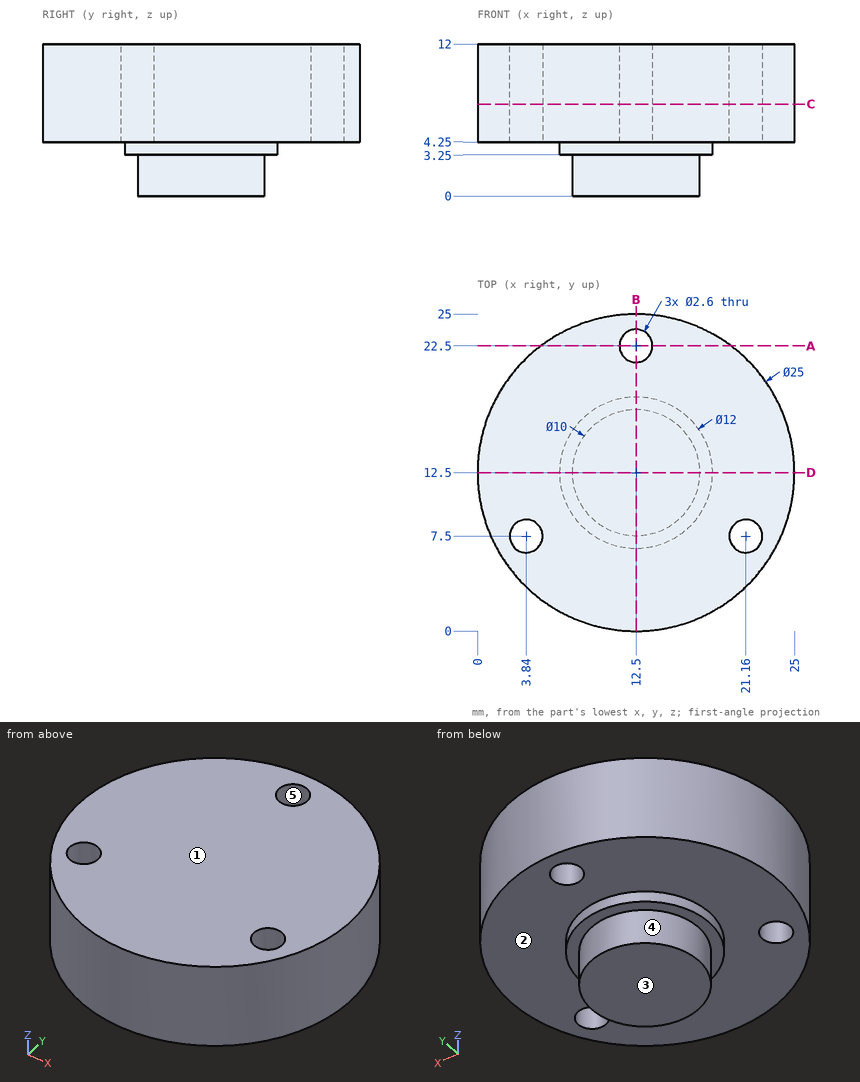
Part print with two shaded views. Sizes in mm from the minimum x, y, z corner. A direction names the side the tool comes from. Round coordinates to 2 decimals unless told otherwise and drop trailing zeros. Order: outer loops, then holes, each group sorted by start corner. A loop starts at its lowest first (then second) coordinate and runs counter-clockwise, first axis right, second up. Notation, with made-up numbers: (2.5, 71) - (56.5, 71) arc R18 ccw to (56.5, 97) - close; hole circle Ø10 at (70, 67.5). An arc over 180 degrees is marked (long way). Answer as CSV lines item,"result". Start each with the question number.
1. Drill centre lines: L1, parallel to Y at x = 12.5, z = 7.75; L2, parallel to Z at x = 15.5, y = 20; L3, parallel to Y at x = 11.5, z = 11.25. Where is each one in solid material? Low to high. Write a range as [from, to].
2. Tool access for the marked faces 1 and 2: list every direction of +Z, -Z, +X, -X, +Y, -Y with a clear straight run to the whole face (end or side of a thin tool).
3. Pin check, flat tips, straight feed: pin 1 (1.5 mm diameter, centred on y = 10, z = 3, fed in from -X); pin 2 (2.5 mm diameter, centred on x = 3.84, y = 7.5, fed in from -Z); pin 3 (1.5 mm diameter, centred on x = 6.5, z = 10.5, fed in from -Y); pin 4 (1.5 mm diameter, centred on x = 17, y = 18.5, fed in from -Z). Stop position of each tip, or through.
4. Saw through at A-A, the plane y = 22.5. Write the cut outline in (x, z).
5. Saw through at D-D, the plane y = 12.5. Write the cut outline in (x, z).
6. Saw through at C-C, the plane z = 7.25. Write the cut outline in (x, y), and give its area (3 significant figures).
7. Pull direction X, two halves, no side cores. Call the marked faces 3, 4 and 5: +X half, -X half, draft (parallel to the pull), parting line (faces both ways), or undercut.
8. Saw through at B-B, the plane x = 12.5. Write the cut outline in (y, z), and give its area (3 significant figures).
Model answer:
1,L1,"y = [0, 21.2], [23.8, 25]"
1,L2,"z = [4.25, 12]"
1,L3,"y = [0.04, 21.67], [23.33, 24.96]"
2,face 1,"+Z, +X, -X, +Y, -Y"
2,face 2,"-Z"
3,pin 1,"stops at x = 6.77"
3,pin 2,"passes through"
3,pin 3,"stops at y = 1.16"
3,pin 4,"stops at z = 4.25"
4,outline,"(5, 4.25) - (11.2, 4.25) - (11.2, 12) - (5, 12) - close; (13.8, 4.25) - (20, 4.25) - (20, 12) - (13.8, 12) - close"
5,outline,"(0, 4.25) - (6.5, 4.25) - (6.5, 3.25) - (7.5, 3.25) - (7.5, 0) - (17.5, 0) - (17.5, 3.25) - (18.5, 3.25) - (18.5, 4.25) - (25, 4.25) - (25, 12) - (0, 12) - close"
6,outline,"circle Ø25 at (12.5, 12.5); hole circle Ø2.6 at (3.84, 7.5); hole circle Ø2.6 at (12.5, 22.5); hole circle Ø2.6 at (21.16, 7.5)"
6,area,"475 mm²"
7,face 3,"draft"
7,face 4,"parting line"
7,face 5,"undercut"
8,outline,"(0, 4.25) - (6.5, 4.25) - (6.5, 3.25) - (7.5, 3.25) - (7.5, 0) - (17.5, 0) - (17.5, 3.25) - (18.5, 3.25) - (18.5, 4.25) - (21.2, 4.25) - (21.2, 12) - (0, 12) - close; (23.8, 4.25) - (25, 4.25) - (25, 12) - (23.8, 12) - close"
8,area,"218 mm²"
